Source: three-view drawing plus pictorial views. Frame: mm from the lowest corner of the part. Round coordinates to 2 decimals unless told otherwise and drop trailing zeros. Loops run counter-clockwise (first coordinate to the right, second up) from the corner with the lowest first, then second, coordinate; pieces in that order, holes last. Notation, with made-up numbers: (86, 48) -> (105, 48) arc R17 ccw to (105, 68) -> close; hole circle Ø6 at (3.5, -19.5). An arc over 180 degrees is marked (long way). Answer in a Markdown table with one row per item.
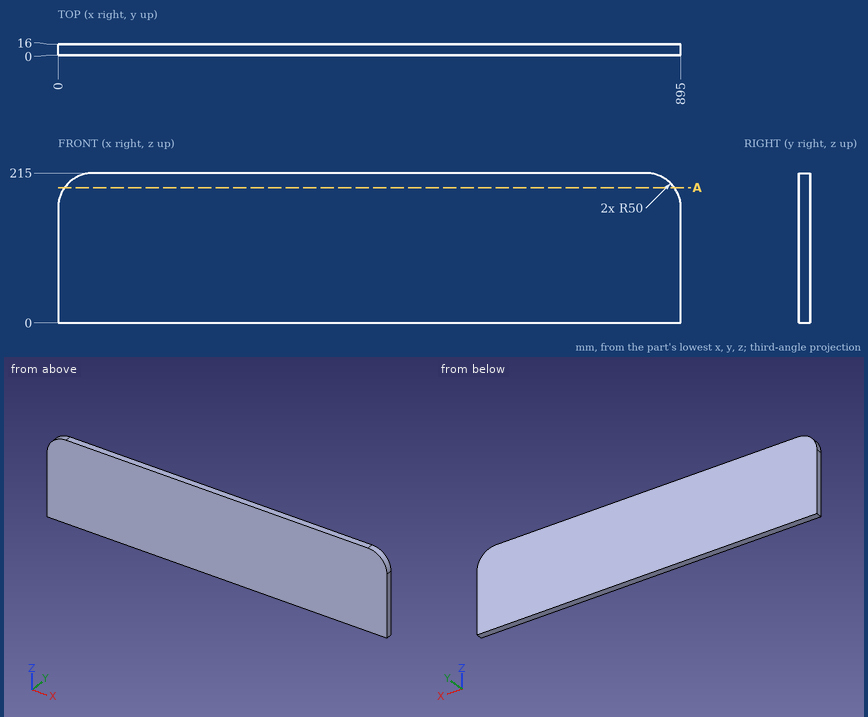
Item 1: Line query: probe 1 along X at (y, z) = (8.5, 198); probe 2 along X at (y, z) = (12.25, 178). Output: solid intervals per line, ascending. Write a range as [from, to].
Answer:
| item | result |
|---|---|
| probe 1 | x = [12.44, 882.56] |
| probe 2 | x = [1.72, 893.28] |
Item 2: Cut plane A-A (z = 194). Output: boundary loops of the cut face in (x, y), then the cut area to 3 significant figures.
Answer:
| item | result |
|---|---|
| outline | (9.27, 0) -> (885.73, 0) -> (885.73, 16) -> (9.27, 16) -> close |
| area | 14,000 mm² |
Item 3: Pin query (flat end, axial travel): pin 1 Ø4 at (x, y) = (773.5, 12) entering from -Z. Return the tip coordinate at first contact, or that it passes through.
Answer:
| item | result |
|---|---|
| pin 1 | stops at z = 0 |
